```python
from build123d import *

# Parameters (mm, degrees)
EXTRUDE_1_DEPTH = 3.9
CHAMFER_1_SIZE  = 1
CHAMFER_1_SIZE2 = 0.577350269


with BuildPart() as part:
    # Эскиз1 → Бобышка-Вытянуть1 (new, symmetric)
    with BuildSketch(Plane(origin=(0, 0, 0), x_dir=(0, 0, -1), z_dir=(1, 0, 0))):
        Polygon((0, 0), (0, 1.5), (2.9, 1.5), (2.9, 0), (4.5, 0), (4.5, -14), (0, -14), align=None)
    extrude(amount=EXTRUDE_1_DEPTH, both=True)

    # Фаска1
    chamfer_1_edges = [part.edges().sort_by_distance(p)[0] for p in [
        (0, -14, 0),
    ]]
    chamfer_1_side = [part.faces().sort_by_distance(p)[0] for p in [
        (0, -6.25, 0),
    ]]
    chamfer(chamfer_1_edges, length=CHAMFER_1_SIZE, length2=CHAMFER_1_SIZE2, reference=chamfer_1_side[0])


solid = part.part
```
Input: part model. Units: mm. Frame: model coordinates. A direction names the side the tool comes from. Give positions to 0.01 mm unless a question says otherwise; leave off trailing zeros. Order: outer loops, then holes, each group sorted by start corner. A loop starts at its lowest first (then second) coordinate and runs counter-clockwise, first axis right, second up. Notation, with made-up numbers: M 58,-36 L 96,-36 A7 cw 96,-27 Z; hole C -34.75,-31 d3. An arc over 180 degrees is marked long. Return JSON: item names as keys, results as strings.
1) Section query A-A on x = 1.25. Output: boundary loops of the cut face in (y, z).
Taken from the geometry:
{"outline": "M -14,-4.5 L 0,-4.5 L 0,-2.9 L 1.5,-2.9 L 1.5,0 L -13,0 L -14,-0.58 Z"}
2) Contact query for flat-ended pins moving along their axis: pin 1 (0.5 mm diameter, centred on x = 0, z = -4, fed in from +Y); pin 2 (1.6 mm diameter, centred on x = 1, y = 1, fed in from -Z). Output: stop coordinate, or through.
Taken from the geometry:
{"pin 1": "stops at y = 0", "pin 2": "stops at z = -2.9"}
3) Section query B-B on y = 0.5. Output: boundary loops of the cut face in (x, z).
Taken from the geometry:
{"outline": "M -3.9,-2.9 L 3.9,-2.9 L 3.9,0 L -3.9,0 Z"}
4) Line query: L1, parallel to Y at x = -1.75, z = -3.15; L2, parallel to Z at x = -2.75, y = 0.5; L3, parallel to Y at x = -3, z = -0.4. Output: solid intervals per line, ascending. Write a range as [from, to].
Taken from the geometry:
{"L1": "y = [-14, 0]", "L2": "z = [-2.9, 0]", "L3": "y = [-13.69, 1.5]"}
5) Section query C-C on z = -3.15. Output: boundary loops of the cut face in (x, y).
Taken from the geometry:
{"outline": "M -3.9,-14 L 3.9,-14 L 3.9,0 L -3.9,0 Z"}
6) Access query for faces 1 (the face through (0, 1, -2.9)), 2 (the face through (0, -14, -3)). Directions: +Z, -Z, +X, -X, +Y, -Y. A direction counts if a zero-diameter tool reaches every point of the face in a straight line with its end or side. Return the directions, or none.
Taken from the geometry:
{"face 1": "-Z, +X, -X, +Y", "face 2": "+Z, -Z, +X, -X, -Y"}
